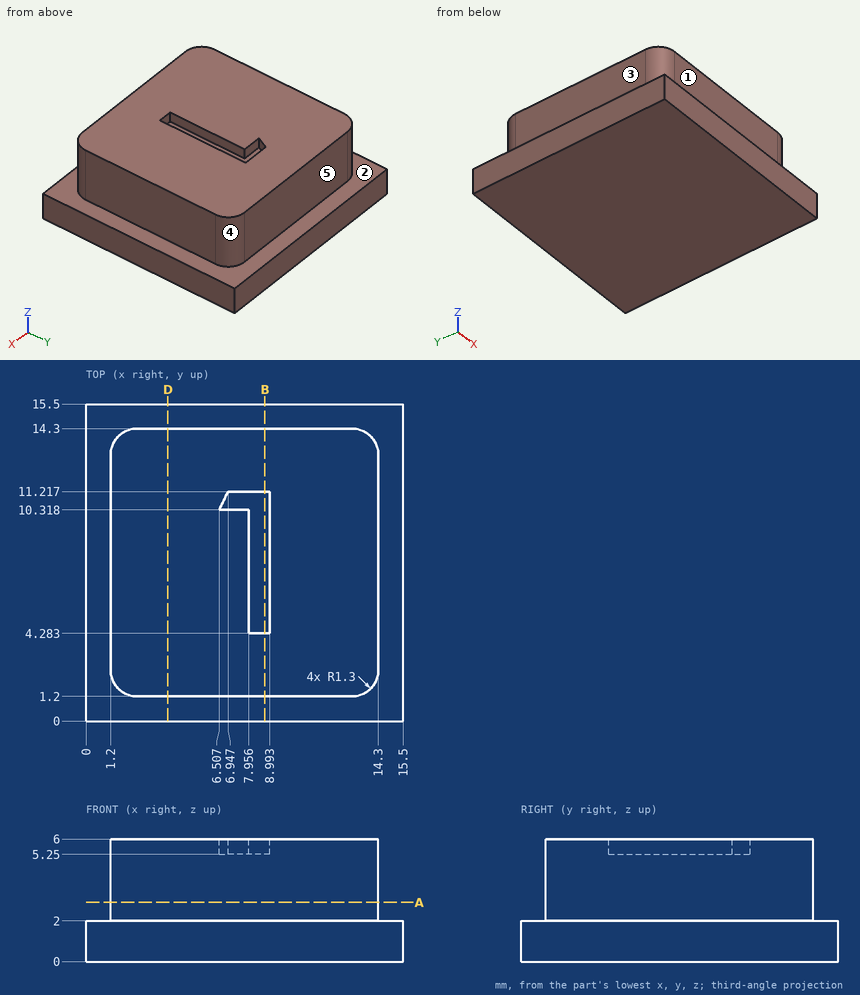
Geometry check sheet. Reference: drawing and pictorial views, mm from the part's lowest x, y, z. A direction names the side the tool comes from. Round coordinates to 2 decimals unless told otherwise and drop trailing zeros. Loops run counter-clockwise (first coordinate to the right, second up) from the corner with the lowest first, then second, coordinate; pieces in that order, holes last. Notation, with made-up numbers: (-3.75, 81.25) -> (4.25, 81.25) arc R28 cw to (4.25, 110.25) -> close; hole circle Ø3 at (16, -21.5). An arc over 180 degrees is marked (long way). Answer as a JSON object with one key per item and string values.
Q1. Section check B-B (x = 8.75). Record the boundary of the cut face in (y, z).
Data:
{"outline": "(0, 0) -> (15.5, 0) -> (15.5, 2) -> (14.3, 2) -> (14.3, 6) -> (11.22, 6) -> (11.22, 5.25) -> (4.28, 5.25) -> (4.28, 6) -> (1.2, 6) -> (1.2, 2) -> (0, 2) -> close"}
Q2. Access from +Z, -Z, +X, -X, +Y, -Y to the whole of each face (thin tool, end or side, straight path). Record for the marked faces 1, 2, 3, 4 and 5.
Data:
{"face 1": "+Z, +X, -X, -Y", "face 2": "+Z", "face 3": "+Z, -X, +Y, -Y", "face 4": "+Z, +X, +Y", "face 5": "+Z, +X, -X, +Y"}
Q3. Go/stop test with flat-tipped pins: P1, Ø0.8, axis at y = 9, z = 5.5, coming from the -X side; P2, Ø3, axis at y = 3.5, z = 2.5, coming from the +X side; P3, Ø3, axis at y = 9.5, z = 4, coming from the +X side; P4, Ø0.8, axis at x = 7.5, z = 5.5, coming from the -Y side. Record where each tip stops, or that it passes through.
Data:
{"P1": "stops at x = 1.2", "P2": "stops at x = 15.5", "P3": "stops at x = 14.3", "P4": "stops at y = 1.2"}
Q4. Section check D-D (x = 4). Record the boundary of the cut face in (y, z).
Data:
{"outline": "(0, 0) -> (15.5, 0) -> (15.5, 2) -> (14.3, 2) -> (14.3, 6) -> (1.2, 6) -> (1.2, 2) -> (0, 2) -> close"}
Q5. Scan lines: line 1 (Y direction, x = 3.5, z = 2.3); line 2 (Z direction, x = 15, y = 1). Record each from-to range of solid material in increasing order. Write a range as from..to.
Data:
{"line 1": "y = 1.2..14.3", "line 2": "z = 0..2"}
Q6. Section check A-A (z = 2.9). Record the boundary of the cut face in (x, y).
Data:
{"outline": "(1.2, 2.5) arc R1.3 ccw to (2.5, 1.2) -> (13, 1.2) arc R1.3 ccw to (14.3, 2.5) -> (14.3, 13) arc R1.3 ccw to (13, 14.3) -> (2.5, 14.3) arc R1.3 ccw to (1.2, 13) -> close"}
